Source: CAD feature listing. Evaluate the final solid. Frame: model axes, mm. A direction names the side the tool comes from. Give positions to 0.01 mm unless a question says otherwise; leave off trailing zeros. Loops run counter-clockwise (first coordinate to the right, second up) from the corner with the lowest first, then second, coordinate; pieces in that order, holes last. Notation, with made-up numbers: (9.5, -11) - (63.5, -11) arc R29 ccw to (63.5, 26) - close; hole circle Ø2 at (28, -0.5). An arc over 180 degrees is marked (long way). Put each result on its own line as item: value.
```python
from build123d import *

# Parameters (mm, degrees)
SKETCH002_R  = 3
PAD002_DEPTH = 22
SKETCH001_R  = 4.5
PAD001_DEPTH = 60
PAD003_DEPTH = 6
PAD_DEPTH    = 80
FILLET_R     = 10


with BuildPart() as motormount:
    # Sketch002 → Pad002 (new body)
    with BuildSketch(Plane(origin=(0, 12.41006, 0), x_dir=(-1, 0, 0), z_dir=(0, 1, 0))):
        with Locations((-23.592787, 58)):
            Circle(SKETCH002_R)
        with Locations((12.407213, 58)):
            Circle(SKETCH002_R)
    extrude(amount=-PAD002_DEPTH)


with BuildPart() as framemount:
    # Sketch001 → Pad001 (new body)
    with BuildSketch(Plane.YZ.offset(35.592787)):
        with Locations((2, 70)):
            Circle(SKETCH001_R)
        with Locations((2, 10)):
            Circle(SKETCH001_R)
    extrude(amount=-PAD001_DEPTH)


with BuildPart() as cutblock:
    # Sketch003 → Pad003 (new body)
    with BuildSketch(Plane(origin=(0, 12.41006, 0), x_dir=(-1, 0, 0), z_dir=(0, 1, 0))):
        Polygon((-20.742787, 53.063655), (-17.892787, 58), (-20.742787, 62.936345), (-26.442787, 62.936345), (-29.292787, 58), (-26.442787, 53.063655), align=None)
        Polygon((15.257213, 53.063655), (18.107213, 58), (15.257213, 62.936345), (9.557213, 62.936345), (6.707213, 58), (9.557213, 53.063655), align=None)
    extrude(amount=-PAD003_DEPTH)

    # Fusion: union MotorMount, FrameMount
    add(motormount.part)
    add(framemount.part)


with BuildPart() as fillet_body:
    # Sketch → Pad (new body)
    with BuildSketch(Plane.XY):
        with BuildLine():
            Line((-24.407213, 12.41006), (35.592787, 12.41006))
            Line((35.592787, 12.41006), (35.592787, -9.58994))
            Line((9.592787, -9.58994), (35.592787, -9.58994))
            ThreePointArc((9.592787, -9.58994), (5.592787, -5.58994), (1.592787, -9.58994))
            Line((-24.407213, -9.58994), (1.592787, -9.58994))
            Line((-24.407213, -9.58994), (-24.407213, 12.41006))
        make_face()
    extrude(amount=PAD_DEPTH)

    # Cut: cut CutBlock
    add(cutblock.part, mode=Mode.SUBTRACT)

    # Fillet
    fillet_edges = [fillet_body.edges().sort_by_distance(p)[0] for p in [
        (5.592787, 12.41006, 80),
        (5.592787, 12.41006, 0),
    ]]
    fillet(fillet_edges, radius=FILLET_R)


solid = fillet_body.part
```
1) Access query for faces 4 (the flat face through (22, -9.59, 39)), 5 (the flat face through (-15, 6.41, 56)). Directions: +Z, -Z, +X, -X, +Y, -Y. A direction counts if a zero-diameter tool reaches every point of the face in a straight line with its end or side. Return the directions, or none.
Check result:
face 4: +Z, -Z, +X, -X, -Y
face 5: +Y
2) Section query D-D, the plane z = 17.5. Output: boundary loops of the cut face in (x, y).
Check result:
outline: (-24.41, -9.59) - (1.59, -9.59) arc R4 cw to (9.59, -9.59) - (35.59, -9.59) - (35.59, 12.41) - (-24.41, 12.41) - close
3) Material intervals for line 1 along Z through (x, y) = (20.5, 2); line 2 along Z through (x, y) = (-3, 5); line 3 along X through (y, z) = (-8, 52), sorted ascending. Write a range as [from, to].
Check result:
line 1: [0, 5.5], [14.5, 65.5], [74.5, 80]
line 2: [0.34, 6.65], [13.35, 66.65], [73.35, 79.66]
line 3: [-24.41, 1.92], [9.26, 35.59]
4) Section query B-B, the plane y = 4.5. Output: boundary loops of the cut face in (x, z).
Check result:
outline: (-24.41, 0.22) - (35.59, 0.22) - (35.59, 6.26) - (-24.41, 6.26) - close; (-24.41, 13.74) - (35.59, 13.74) - (35.59, 66.26) - (-24.41, 66.26) - close; (-24.41, 73.74) - (35.59, 73.74) - (35.59, 79.78) - (-24.41, 79.78) - close; hole circle Ø6 at (-12.41, 58); hole circle Ø6 at (23.59, 58)
5) Pin query (flat end, axial travel): P1, Ø3, axis at x = -11, y = 8, coming from the -Z side; P2, Ø9.5, axis at x = -12.41, z = 58, coming from the +Y side; P3, Ø1.7, axis at x = -11.5, y = 9, coming from the +Z side. Return the tip coordinate at first contact, or that it passes through.
Check result:
P1: z = 0.87
P2: y = 6.41
P3: z = 78.19
6) Section query A-A, the plane x = 15. Output: boundary loops of the cut face in (y, z), plus the area to 3 significant figures.
Check result:
outline: (-9.59, 0) - (2.41, 0) arc R10 ccw to (12.41, 10) - (12.41, 70) arc R10 ccw to (2.41, 80) - (-9.59, 80) - close; hole circle Ø9 at (2, 10); hole circle Ø9 at (2, 70)
area: 1,590 mm²
7) Section query C-C, the plane y = 0.5. Output: boundary loops of the cut face in (x, z).
Check result:
outline: (-24.41, 0) - (35.59, 0) - (35.59, 5.76) - (-24.41, 5.76) - close; (-24.41, 14.24) - (35.59, 14.24) - (35.59, 65.76) - (-24.41, 65.76) - close; (-24.41, 74.24) - (35.59, 74.24) - (35.59, 80) - (-24.41, 80) - close; hole circle Ø6 at (-12.41, 58); hole circle Ø6 at (23.59, 58)
8) Mould query, pull axis X, two halves, no side actions, for faces 1 (the cylindrical face through (6.01, 9.56, 3.01)), 2 (the flat face through (-12, 9, 62.936)), 3 (the flat face through (35.593, 2, 39)). Classes: pulls with the +X half, pulls with the -X half, needs draft (parallel to the pull), parting line crosses it, or undercut.
Check result:
face 1: needs draft
face 2: undercut
face 3: pulls with the +X half
